```python
from build123d import *

# Parameters (mm, degrees)
CYLINDER188_R          = 2
CYLINDER188_DEPTH      = 13
CYLINDER187_R          = 2
CYLINDER187_DEPTH      = 13
BOX321_W               = 23
BOX321_H               = 5
BOX321_DEPTH           = 25
BOX098_W               = 35
BOX098_H               = 5
BOX098_DEPTH           = 25
BOX097_W               = 52
BOX097_H               = 5
BOX097_DEPTH           = 25
CUT144_PLACEMENT_ANGLE = 90


with BuildPart() as cylinder188:
    # Cylinder188 → Cylinder188 (new body)
    with BuildSketch(Plane(origin=(-12, -69, -5), x_dir=(1, 0, 0), z_dir=(0, 0, 1))):
        Circle(CYLINDER188_R)
    extrude(amount=CYLINDER188_DEPTH)


with BuildPart() as cylinder187:
    # Cylinder187 → Cylinder187 (new body)
    with BuildSketch(Plane(origin=(-55, -69, -5), x_dir=(1, 0, 0), z_dir=(0, 0, 1))):
        Circle(CYLINDER187_R)
    extrude(amount=CYLINDER187_DEPTH)


with BuildPart() as box321:
    # Box321 → Box321 (new body)
    with BuildSketch(Plane(origin=(-46, -93, 16), x_dir=(1, 0, 0), z_dir=(0, 0, 1))):
        with Locations((11.5, 2.5)):
            Rectangle(BOX321_W, BOX321_H)
    extrude(amount=BOX321_DEPTH)


with BuildPart() as box098:
    # Box098 → Box098 (new body)
    with BuildSketch(Plane(origin=(-52, -88, 16), x_dir=(1, 0, 0), z_dir=(0, 0, 1))):
        with Locations((17.5, 2.5)):
            Rectangle(BOX098_W, BOX098_H)
    extrude(amount=BOX098_DEPTH)


with BuildPart() as cut148:
    # Box097 → Box097 (new body)
    with BuildSketch(Plane(origin=(-60, -93, 16), x_dir=(1, 0, 0), z_dir=(0, 0, 1))):
        with Locations((26, 2.5)):
            Rectangle(BOX097_W, BOX097_H)
    extrude(amount=BOX097_DEPTH)

    # Fusion: union Box098
    add(box098.part)

    # Cut144: cut Box321
    add(box321.part, mode=Mode.SUBTRACT)


with BuildPart() as cut148_1:
    # Cut144 placement: moved
    add(cut148.part.moved(Location((0, -40, 96))).rotate(Axis((0, -40, 96), (1, 0, 0)), CUT144_PLACEMENT_ANGLE))

    # Cut147: cut Cylinder187
    add(cylinder187.part, mode=Mode.SUBTRACT)

    # Cut148: cut Cylinder188
    add(cylinder188.part, mode=Mode.SUBTRACT)


with BuildPart() as cut148_2:
    # Cut148 placement: moved
    add(cut148_1.part.moved(Location((0, 8, 42))))


solid = cut148_2.part
```
Source: CAD feature listing. Evaluate the final solid. Frame: model axes, mm. A direction names the side the tool comes from. Coordinates: 2 decimals unless noted, no trailing zeros. Order: outer loops, then holes, each group sorted by start corner. A loop starts at its lowest first (then second) coordinate and runs counter-clockwise, first axis right, second up. Notation, with made-up numbers: M 76,49.25 L 98,49.25 A18 ccw 98,54.25 Z; hole C -15.5,28 d9. An arc over 180 degrees is marked long. Write each question's results on one line, items separated by ' | '. Start each with the question number.
1) Section query B-B (x = -12). Return the cut outline in (y, z), plus the area to 3 significant figures.
2) Contact query for flat-ended pins moving along their axis: pin 1 Ø5 at (x, y) = (-12, -61) entering from -Z; pin 2 Ø1.5 at (x, y) = (-37, -56.5) entering from -Z; pin 3 Ø1.5 at (y, z) = (-54.5, 53.5) entering from -X; pin 4 Ø4 at (x, y) = (-54.5, -65.5) entering from +Z. Output: stop coordinate, or through.
3) Section query D-D (z = 51.75). Return the cut outline in (x, y).
4) Section query C-C (y = -61). Return the cut outline in (x, z).
5) Line query: line 1 (X direction, y = -61, z = 46.95); line 2 (Y direction, x = -55, z = 48.65); line 3 (X direction, y = -56.75, z = 47.25). Output: solid intervals per line, ascending. Write a range as from..to.
6) Draft query along Y for faces 1 (the face through (-53.925, -59.314, 47.465)), 2 (the face through (-34, -73, 51)), 3 (the face through (-46, -60, 47)). Return one class per face: released by +Y, released by -Y, zero draft, split by the parting line, or undercut.
7) Section query A-A (z = 48). Return the cut outline in (x, y), plus the area to 3 significant figures.
8) Access query for faces 4 (the face through (-17, -60, 52)), 5 (the face through (-23, -60, 47)), 6 (the face through (-52, -60, 52)). Directions: +Z, -Z, +X, -X, +Y, -Y. A direction counts if a zero-diameter tool reaches every point of the face in a straight line with its end or side. Return the directions, or none.
Answers:
1) outline: M -73,45 L -63,45 L -63,50 L -73,50 Z; M -59,45 L -48,45 L -48,50 L -59,50 Z | area: 105 mm^2
2) pin 1: stops at z = 45 | pin 2: stops at z = 50 | pin 3: stops at x = -52 | pin 4: stops at z = 50
3) outline: M -52,-73 L -17,-73 L -17,-48 L -52,-48 Z
4) outline: M -60,45 L -57,45 L -57,50 L -60,50 Z; M -53,45 L -46,45 L -46,50 L -23,50 L -23,45 L -14,45 L -14,50 L -17,50 L -17,55 L -52,55 L -52,50 L -53,50 Z; M -10,45 L -8,45 L -8,50 L -10,50 Z
5) line 1: x = -60..-57, -53..-46, -23..-14, -10..-8 | line 2: y = -73..-63, -59..-48 | line 3: x = -60..-46, -23..-8
6) face 1: undercut | face 2: released by -Y | face 3: zero draft
7) outline: M -60,-73 L -46,-73 L -46,-48 L -60,-48 Z; M -23,-73 L -8,-73 L -8,-48 L -23,-48 Z; hole C -55,-61 d4; hole C -12,-61 d4 | area: 700 mm^2
8) face 4: +Z, +X, +Y, -Y | face 5: -Z, +Y, -Y | face 6: +Z, -X, +Y, -Y
